Build history of the part. All positions in model axes, mm. A direction names the side the tool comes from. Round coordinates to 2 decimals unless told otherwise and drop trailing zeros. Loops run counter-clockwise (first coordinate to the right, second up) from the corner with the lowest first, then second, coordinate; pieces in that order, holes last. Notation, with made-up numbers: (70, 54) - (110, 54) arc R20 cw to (110, 76) - close; hole circle Ø6 at (-36, 83). An arc over 180 degrees is marked (long way). Use one line per item in the form item = value. Start each with the question number.
Q1. Saw through at C-C (x = -37.75). Give the cut face in (y, z).
Q2. Pin check, flat tips, straight feed: pin 1 (2 mm diameter, centred on x = -38.35, y = 34.82, fed in from +Z); pin 2 (5 mm diameter, centred on y = 31.5, z = -3.5, fed in from +X); pin 3 (5.5 mm diameter, centred on x = -29, y = 25.47, fed in from +Z); pin 4 (6 mm diameter, centred on y = 28.5, z = 7, fed in from +X). Stop position of each tip, or through.
Q3. Saw through at D-D (y = 32.75). Count the separate pieces of the cut face and the enclosed holes in it, then the cut area to 3 significant figures.
Q4. Mould opens along X. For faces 5 (the face through (-44.55, 25.2, -3.3)), 6 (the face through (-42.5, 29.6, 0)), 7 (the face through (-36.368, 24.648, 3.123)), 8 (the face through (-38, 25, -6.7)) say: released by +X, released by -X, zero draft, split by the parting line, or undercut.
Q5. Saw through at A-A (x = -28.5). Give the cut face in (y, z).
Q6. Saw through at B-B (z = 4). Give the cut face in (x, y), then the cut area to 3 significant figures.
Q7. 3-axis set-ups, long thin cutter, end or side, ignore diameter. For faces 1 (the face through (-38, 26, -3.95)), 2 (the face through (-35, 20, 0)), 3 (the face through (-44.701, 33.937, 2.934)), 4 (the face through (-45.58, 28.31, 3.04)): which of +Z, -Z, +X, -X, +Y, -Y reach the whole face in a straight line?
Q8. Drill centre lines: line 1 (X direction, y = 24, z = 3.5); line 2 (Y direction, x = -37.75, z = 5.25); line 3 (Z direction, x = -44.25, y = 14.75). Where is each one in solid material? Low to high.
```python
from build123d import *

# Parameters (mm, degrees)
ESBO_O1_R                         = 12.5
RESSALTO_EXTRUS_O1_DEPTH          = 6
ESBO_O5_R                         = 6.2
RESSALTO_EXTRUS_O2_DEPTH          = 6.7
ESBO_O6_R                         = 5.7
RESSALTO_EXTRUS_O3_DEPTH          = 4
ESBO_O7_R                         = 2.15
CORTE_EXTRUS_O1_DEPTH             = 13.95
ESBO_O10_R                        = 1.75
CORTE_EXTRUS_O2_DEPTH             = 65.724771281
CORTE_EXTRUS_O3_DEPTH             = 6
CORTE_EXTRUS_O4_REACH             = 31.83
ESBO_O12_R                        = 1.5
CORTE_EXTRUS_O4_DIRECTION_2_REACH = 31.83


with BuildPart() as part:
    # Esboço1 → Ressalto-extrusão1 (new body)
    with BuildSketch(Plane.XY):
        with Locations(Location((-38.354525113, 25.471348315, 0), (0, 0, 180))):
            Circle(ESBO_O1_R)
    extrude(amount=RESSALTO_EXTRUS_O1_DEPTH)

    # Esboço5 → Ressalto-extrusão2 (add)
    with BuildSketch(Plane(origin=(0, 0, 0), x_dir=(-1, 0, 0), z_dir=(0, 0, -1))):
        with Locations(Location((38.354525113, 25.471348315, 0), (0, 0, 180))):
            Circle(ESBO_O5_R)
    extrude(amount=RESSALTO_EXTRUS_O2_DEPTH)

    # Esboço6 → Ressalto-extrusão3 (add)
    with BuildSketch(Plane.XY.offset(6)):
        with Locations((-38.354525113, 25.471348315)):
            Circle(ESBO_O6_R)
    extrude(amount=RESSALTO_EXTRUS_O3_DEPTH)

    # Esboço7 → Corte-extrusão1 (cut)
    with BuildSketch(Plane.XY.offset(10)):
        with Locations((-38.354525113, 25.471348315)):
            Circle(ESBO_O7_R)
    extrude(amount=-CORTE_EXTRUS_O1_DEPTH, mode=Mode.SUBTRACT)

    # Esboço10 → Corte-extrusão2 (cut, through all)
    with BuildSketch(Plane.XY.offset(6)):
        with Locations((-38.354525113, 34.821348315)):
            Circle(ESBO_O10_R)
        with Locations((-38.354525113, 16.121348315)):
            Circle(ESBO_O10_R)
        with Locations((-29.004525113, 25.471348315)):
            Circle(ESBO_O10_R)
        with Locations((-47.704525113, 25.471348315)):
            Circle(ESBO_O10_R)
    extrude(amount=-CORTE_EXTRUS_O2_DEPTH, mode=Mode.SUBTRACT)

    # Esboço9 → Corte-extrusão3 (cut)
    with BuildSketch(Plane.XY.offset(6)):
        Polygon((-44.577064788, 27.309825946), (-40.193002744, 31.693887989), (-42.172901732, 33.673786976), (-46.556963775, 29.289724933), align=None)
    extrude(amount=-CORTE_EXTRUS_O3_DEPTH, mode=Mode.SUBTRACT)

    # Esboço12 → Corte-extrusão4 (cut, up to next)
    with BuildSketch(Plane(origin=(-37.923344354, 37.923344354, 0), x_dir=(0, 0, -1), z_dir=(0.7071067811865457, -0.7071067811865493, 0)), mode=Mode.PRIVATE) as corte_extrus_o4_sk1:
        with Locations(Location((-3, -9.109781678, 0), (0, 0, 270))):
            Circle(ESBO_O12_R)
    corte_extrus_o4_tool1 = extrude(corte_extrus_o4_sk1.sketch, amount=-CORTE_EXTRUS_O4_REACH, mode=Mode.PRIVATE) & part.part
    add(corte_extrus_o4_tool1.solids().sort_by_distance((-44.364933, 31.481756, 3))[0], mode=Mode.SUBTRACT)

    # Esboço12 → Corte-extrusão4 direction 2 (cut, up to next)
    with BuildSketch(Plane(origin=(-37.923344354, 37.923344354, 0), x_dir=(0, 0, -1), z_dir=(0.7071067811865457, -0.7071067811865493, 0)), mode=Mode.PRIVATE) as corte_extrus_o4_direction_2_sk1:
        with Locations(Location((-3, -9.109781678, 0), (0, 0, 270))):
            Circle(ESBO_O12_R)
    corte_extrus_o4_direction_2_tool1 = extrude(corte_extrus_o4_direction_2_sk1.sketch, amount=CORTE_EXTRUS_O4_DIRECTION_2_REACH, mode=Mode.PRIVATE) & part.part
    add(corte_extrus_o4_direction_2_tool1.solids().sort_by_distance((-44.364933, 31.481756, 3))[0], mode=Mode.SUBTRACT)


solid = part.part
```
Report:
q1.outline = (12.99, 0) - (14.48, 0) - (14.48, 6) - (12.99, 6) - close; (17.76, 0) - (19.3, 0) - (19.3, -6.7) - (31.64, -6.7) - (31.64, 0) - (33.18, 0) - (33.18, 6) - (31.14, 6) - (31.14, 10) - (27.53, 10) - (27.53, -3.95) - (23.41, -3.95) - (23.41, 10) - (19.8, 10) - (19.8, 6) - (17.76, 6) - close; (36.46, 0) - (37.96, 0) - (37.96, 6) - (36.46, 6) - close
q2.pin_1 = through
q2.pin_2 = -33.26
q2.pin_3 = 6
q2.pin_4 = -25.86
q3.separate_pieces = 2
q3.enclosed_holes = 1
q3.area = 101 mm²
q4.face_5 = split by the parting line
q4.face_6 = undercut
q4.face_7 = undercut
q4.face_8 = zero draft
q5.outline = (17.78, 0) - (23.8, 0) - (23.8, 6) - (17.78, 6) - close; (27.15, 0) - (33.16, 0) - (33.16, 6) - (27.15, 6) - close
q6.outline = (-47.95, 33.48) arc R12.5 ccw (long way) to (-46.37, 35.07) - (-43.57, 32.27) - (-42.17, 33.67) - (-40.19, 31.69) - (-41.59, 30.29) - (-38.86, 27.56) arc R2.15 cw (long way) to (-40.44, 25.98) - (-43.18, 28.71) - (-44.58, 27.31) - (-46.56, 29.29) - (-45.16, 30.69) - close; hole circle Ø3.5 at (-47.7, 25.47); hole circle Ø3.5 at (-38.35, 16.12); hole circle Ø3.5 at (-38.35, 34.82); hole circle Ø3.5 at (-29, 25.47)
q6.area = 403 mm²
q7.face_1 = +Z
q7.face_2 = -Z
q7.face_3 = none
q7.face_4 = +Z, -Z
q8.line_1 = -50.77 to -48.65, -46.76 to -39.92, -36.79 to -29.95, -28.06 to -25.94
q8.line_2 = 12.99 to 14.48, 17.76 to 23.41, 27.53 to 33.18, 36.46 to 37.96
q8.line_3 = 0 to 6
